Drawing for the job (mm, zero at the part's lowest x, y, z). Round coordinates to 2 decimals unless told otherwise and drop trailing zeros. Order: outer loops, then holes, each group sorted by start corner. A loop starts at its lowest first (then second) coordinate and runs counter-clockwise, first axis right, second up. Notation, with made-up numbers: (36.5, -7.5) -> (71.5, -7.5) arc R13 ccw to (71.5, 10.5) -> close; hole circle Ø3 at (43.25, -36.5). An arc over 180 degrees is marked (long way). Use CSV: the item, a comma, the result in double quotes.
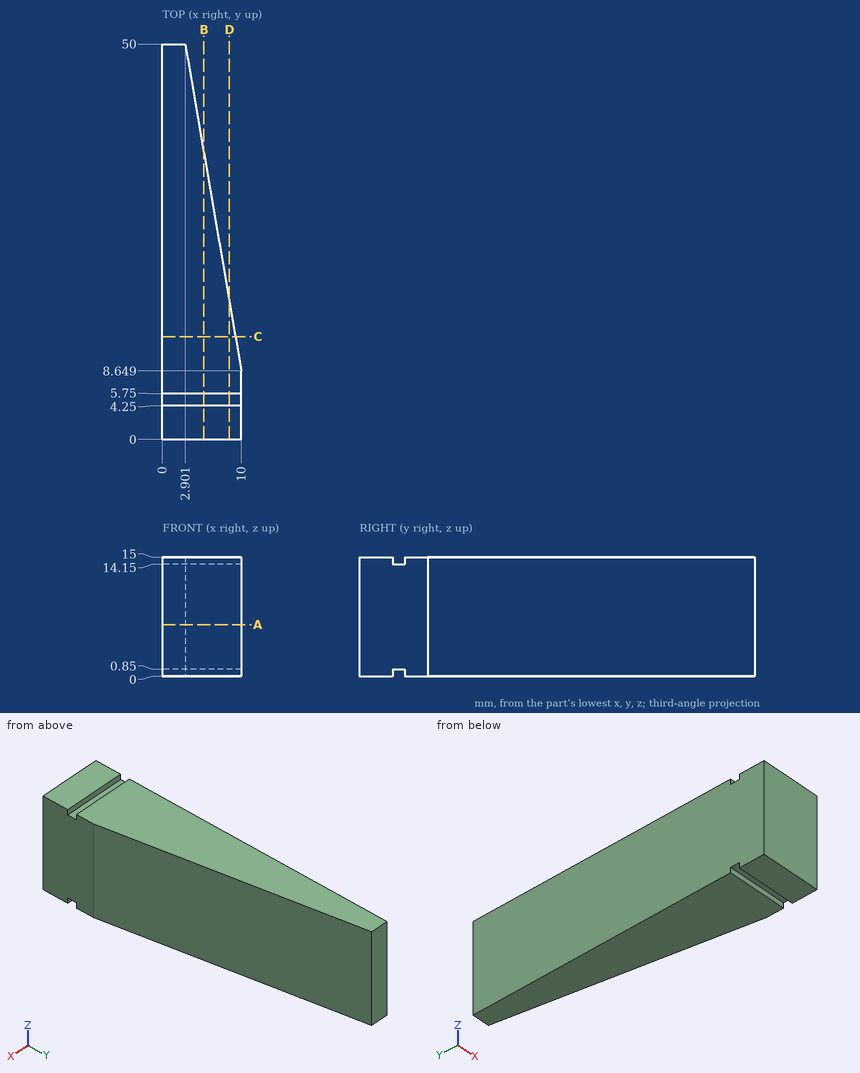
Q1. Probe line 1 along X through (y, z) = (11, 6); line 2 along X through (y, z) = (36.5, 12). List the from-to ranges inside material, lowest first.
From the geometry:
line 1,"x = 0 to 9.6"
line 2,"x = 0 to 5.22"
Q2. Pin check, flat tips, straight feed: pin 1 (0.8 mm diameter, centred on x = 6, y = 5, fed in from -Z); pin 2 (5 mm diameter, centred on y = 32, z = 1.5, fed in from +X); pin 3 (3 mm diameter, centred on x = 8.5, y = 34, fed in from -Z); pin 4 (2 mm diameter, centred on y = 33, z = 13, fed in from +X). Stop position of each tip, or through.
From the geometry:
pin 1,"stops at z = 0.85"
pin 2,"stops at x = 6.42"
pin 3,"passes through"
pin 4,"stops at x = 5.99"
Q3. Cut at A-A (z = 6.5). Give the cut face in (x, y), plus the area to 3 significant figures.
From the geometry:
outline,"(0, 0) -> (10, 0) -> (10, 8.65) -> (2.9, 50) -> (0, 50) -> close"
area,"353 mm²"
Q4. Cut at C-C (y = 13). Give the cut face in (x, z), plus the area to 3 significant figures.
From the geometry:
outline,"(0, 0) -> (9.25, 0) -> (9.25, 15) -> (0, 15) -> close"
area,"139 mm²"
Q5. Cut at D-D (x = 8.5). Give the cut face in (y, z).
From the geometry:
outline,"(0, 0) -> (4.25, 0) -> (4.25, 0.85) -> (5.75, 0.85) -> (5.75, 0) -> (17.39, 0) -> (17.39, 15) -> (5.75, 15) -> (5.75, 14.15) -> (4.25, 14.15) -> (4.25, 15) -> (0, 15) -> close"
Q6. Cut at B-B (x = 5.25). Give the cut face in (y, z), plus the area to 3 significant figures.
From the geometry:
outline,"(0, 0) -> (4.25, 0) -> (4.25, 0.85) -> (5.75, 0.85) -> (5.75, 0) -> (36.32, 0) -> (36.32, 15) -> (5.75, 15) -> (5.75, 14.15) -> (4.25, 14.15) -> (4.25, 15) -> (0, 15) -> close"
area,"542 mm²"
